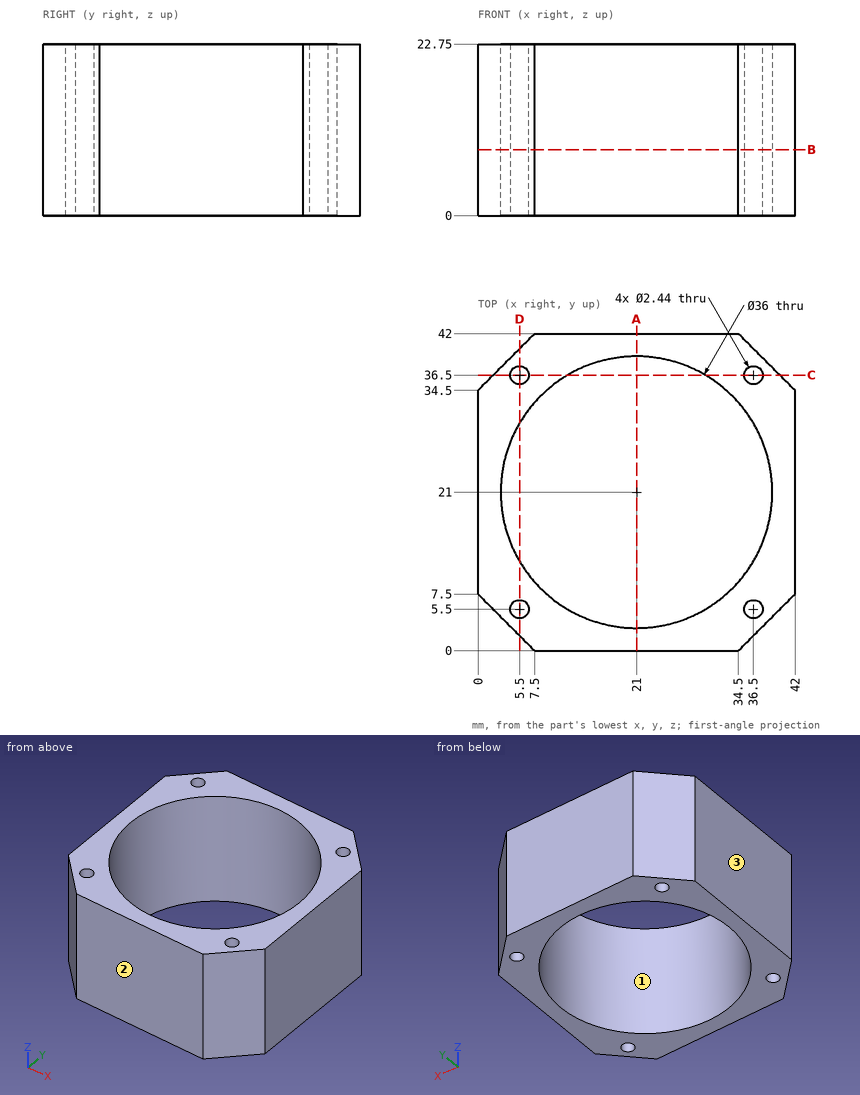
Part print with two shaded views. Sizes in mm from the minimum x, y, z corner. Round coordinates to 2 decimals unless told otherwise and drop trailing zeros. Order: outer loops, then holes, each group sorted by start corner. A loop starts at its lowest first (then second) coordinate and runs counter-clockwise, first axis right, second up. Notation, with made-up numbers: M 61.5,-28 L 87.5,-28 A11 ccw 87.5,-18 Z; hole C 13.5,5 d5. An arc over 180 degrees is marked long. Answer in a Markdown table with one row per item. Add a question column.
Q1. Mould opens along Y. For the marked faces 1, 2 and 3 say: +Y half, -Y half, draft (parallel to the pull), parting line (faces both ways), or undercut.
Q2. Cut at A-A on x = 21. Give the cut face in (y, z).
Q3. Cut at C-C on y = 36.5. Give the cut face in (x, z), and give its area (3 significant figures).
Q4. Cut at B-B on z = 8.75. Give the cut face in (x, y), and give its area (3 significant figures).
Q5. Wall check: L1, parallel to Y at x = 5.5, z = 11.25; L2, parallel to Y at x = 32.5, z = 8.75. Give the ranges that are in metal, low to high. Write a range as from..to.
Q6. Pin check, flat tip, straight feed: pin 1 (4 mm diameter, centred on x = 37, z = 3, fed in from -Y). Stop position of the tip, or through.
Established:
| question | item | result |
|---|---|---|
| 1 | face 1 | undercut |
| 1 | face 2 | -Y half |
| 1 | face 3 | draft |
| 2 | outline | M 0,0 L 3,0 L 3,22.75 L 0,22.75 Z; M 39,0 L 42,0 L 42,22.75 L 39,22.75 Z |
| 3 | outline | M 2,0 L 4.28,0 L 4.28,22.75 L 2,22.75 Z; M 6.72,0 L 11.85,0 L 11.85,22.75 L 6.72,22.75 Z; M 30.15,0 L 35.28,0 L 35.28,22.75 L 30.15,22.75 Z; M 37.72,0 L 40,0 L 40,22.75 L 37.72,22.75 Z |
| 3 | area | 337 mm2 |
| 4 | outline | M 0,7.5 L 7.5,0 L 34.5,0 L 42,7.5 L 42,34.5 L 34.5,42 L 7.5,42 L 0,34.5 Z; hole C 21,21 d36; hole C 5.5,5.5 d2.44; hole C 5.5,36.5 d2.44; hole C 36.5,5.5 d2.44; hole C 36.5,36.5 d2.44 |
| 4 | area | 615 mm2 |
| 5 | L1 | y = 2..4.28, 6.72..11.85, 30.15..35.28, 37.72..40 |
| 5 | L2 | y = 0..7.15, 34.85..42 |
| 6 | pin 1 | stops at y = 0.5 |
